The model under review builds one solid part; all positions refer to its coordinate system, in mm. A direction names the side the tool comes from. Give positions to 0.01 mm unless a question says otherwise; leave off trailing zeros. Loops run counter-clockwise (first coordinate to the right, second up) from the corner with the lowest first, then second, coordinate; pieces in that order, holes last. Notation, with made-up numbers: (5.25, -37) - (25.25, -37) arc R7 cw to (25.25, -29) - close; hole circle Ø6 at (82, -28.5). An arc over 180 degrees is marked (long way). Return JSON: item names as keys, results as strings. Group by question number.
from build123d import *

# Parameters (mm, degrees)
SKETCH1_R           = 4.7625
SKETCH1_R_2         = 1.65
BOSS_EXTRUDE1_DEPTH = 15
SKETCH2_R           = 4.7625
BOSS_EXTRUDE2_DEPTH = 15
CUT_EXTRUDE1_REACH  = 66.755
SKETCH3_R           = 2


with BuildPart() as part:
    # Sketch1 → Boss-Extrude1 (new body, symmetric)
    with BuildSketch(Plane.XY):
        with BuildLine():
            Line((-13.253372163, -1.044486042), (-7.531237528, -10.955513958))
            ThreePointArc((-7.531237528, -10.955513958), (-6.784217233, -11.816359568), (-5.770008435, -12.336431676))
            Line((-5.770008435, -12.336431676), (-0.836847118, -13.76941319))
            ThreePointArc((-0.836847118, -13.76941319), (0, -13.888495471), (0.836847118, -13.76941319))
            Line((0.836847118, -13.76941319), (5.770008435, -12.336431676))
            ThreePointArc((5.770008435, -12.336431676), (6.784217233, -11.816359568), (7.531237528, -10.955513958))
            Line((7.531237528, -10.955513958), (13.253372163, -1.044486042))
            ThreePointArc((13.253372163, -1.044486042), (13.625376182, 0.032875315), (13.568667441, 1.171241953))
            Line((13.568667441, 1.171241953), (12.343085176, 6.159975731))
            ThreePointArc((12.343085176, 6.159975731), (12.027789898, 6.944247736), (11.506238058, 7.609437458))
            Line((11.506238058, 7.609437458), (7.798659006, 11.165189723))
            ThreePointArc((7.798659006, 11.165189723), (6.841158949, 11.783484253), (5.722134635, 12))
            Line((5.722134635, 12), (-5.722134635, 12))
            ThreePointArc((-5.722134635, 12), (-6.841158949, 11.783484253), (-7.798659006, 11.165189723))
            Line((-7.798659006, 11.165189723), (-11.506238058, 7.609437458))
            ThreePointArc((-11.506238058, 7.609437458), (-12.027789898, 6.944247736), (-12.343085176, 6.159975731))
            Line((-12.343085176, 6.159975731), (-13.568667441, 1.171241953))
            ThreePointArc((-13.568667441, 1.171241953), (-13.625376182, 0.032875315), (-13.253372163, -1.044486042))
        make_face()
        Circle(SKETCH1_R, mode=Mode.SUBTRACT)
        with Locations((-8.238066653, 4.75625)):
            Circle(SKETCH1_R_2, mode=Mode.SUBTRACT)
        with Locations((8.238066653, 4.75625)):
            Circle(SKETCH1_R_2, mode=Mode.SUBTRACT)
        with Locations((0, -9.5125)):
            Circle(SKETCH1_R_2, mode=Mode.SUBTRACT)
    extrude(amount=BOSS_EXTRUDE1_DEPTH, both=True)

    # Sketch2 → Boss-Extrude2 (add, symmetric)
    with BuildSketch(Plane.XY):
        with BuildLine():
            Line((-12.421472807, 5.666457921), (-9.735682804, 41.826981922))
            ThreePointArc((-9.735682804, 41.826981922), (0, 50.866372944), (9.735682804, 41.826981922))
            Line((9.735682804, 41.826981922), (12.421472807, 5.666457921))
            Line((12.421472807, 5.666457921), (0, 12))
            Line((0, 12), (-12.421472807, 5.666457921))
        make_face()
        with Locations((0, 41.103872944)):
            Circle(SKETCH2_R, mode=Mode.SUBTRACT)
    extrude(amount=BOSS_EXTRUDE2_DEPTH, both=True)

    # Sketch3 → Cut-Extrude1 (cut, up to next)
    with BuildSketch(Plane(origin=(0, 50.866372944, 0), x_dir=(1, 0, 0), z_dir=(0, 1, 0)), mode=Mode.PRIVATE) as cut_extrude1_sk1:
        Circle(SKETCH3_R)
    cut_extrude1_tool1 = extrude(cut_extrude1_sk1.sketch, amount=-CUT_EXTRUDE1_REACH, mode=Mode.PRIVATE) & part.part
    add(cut_extrude1_tool1.solids().sort_by_distance((0, 50.866373, 0))[0], mode=Mode.SUBTRACT)


solid = part.part
Item 1: Take a section at A-A (x = 0). State the section outline as (y, z) points.
Item 2: For P1, Ø5, axis at x = 9.5, z = -1, coming from the +Y side; P2, Ø2, axis at y = 20, z = 7, coming from the +X side; P3, Ø5, axis at x = 1, z = 10, coming from the -Y side; P4, Ø1, axis at y = 26, z = 4, coming from the -X side, all flat-tipped, find the tip position at first contact; note any pin that passes through.
Item 3: For L1, parallel to Y at x = 0, z = 3.5; L2, parallel to Z at x = 0, y = 49.25; L3, parallel to Y at x = 1, z = 11, list the stretches that pass through material, from the lowest coordinate up. Write a range as from..to.
Item 4: Take a section at B-B (z = 0). State how many separate pieces and enclosed holes the cut face has, then the cut area to 3 significant figures.
Item 5: Take a section at D-D (y = 40). State the section outline as (x, z) points, then the cut area to 3 significant figures.
Item 6: Mouldability with a two-part tool opening along Y and no side actions: class faces 3 (the face through (-3.78, -2.9, -0.21)), 4 (the face through (0, 19, 15)), 5 (the face through (-12.978, 3.577, 0.21)) as +Y half, -Y half, draft (parallel to the pull), parting line (faces both ways), or undercut.
Item 7: Tool access review of faces 1 (the face through (13.623, 0.017, 0.21)), 2 (the face through (0, 48, -2)): name each direction out of +Z, -Z, +X, -X, +Y, -Y from which nothing blocks a thin tool from reaching the whole face with its end or side.
Item 8: Take a section at C-C (x = 8.25). State the section outline as (y, z) points, then the cut area to 3 significant figures.
Check sheet entries:
{
 "1": {"outline": "(-13.89, -15) - (-11.16, -15) - (-11.16, 15) - (-13.89, 15) - close; (-7.86, -15) - (-4.76, -15) - (-4.76, 15) - (-7.86, 15) - close; (4.76, -15) - (36.34, -15) - (36.34, 15) - (4.76, 15) - close; (45.87, -15) - (50.87, -15) - (50.87, -2) - (45.87, -2) - close; (45.87, 2) - (50.87, 2) - (50.87, 15) - (45.87, 15) - close"},
 "2": {"P1": "stops at y = 47.91", "P2": "stops at x = 11.43", "P3": "stops at y = -13.89", "P4": "stops at x = -10.95"},
 "3": {"L1": "y = -13.89..-11.16, -7.86..-4.76, 4.76..36.34, 45.87..50.87", "L2": "z = -15..-2, 2..15", "L3": "y = -13.72..-10.82, -8.2..-4.66, 4.66..36.45, 45.76..50.82"},
 "4": {"separate pieces": "1", "enclosed holes": "4", "area": "1,160 mm^2"},
 "5": {"outline": "(-9.87, -15) - (-4.63, -15) - (-4.63, 15) - (-9.87, 15) - close; (4.63, -15) - (9.87, -15) - (9.87, 15) - (4.63, 15) - close", "area": "314 mm^2"},
 "6": {"face 3": "undercut", "face 4": "draft", "face 5": "+Y half"},
 "7": {"face 1": "+Z, -Z, +X", "face 2": "+Y"},
 "8": {"outline": "(-9.71, -15) - (3.11, -15) - (3.11, 15) - (-9.71, 15) - close; (6.41, -15) - (46.32, -15) - (46.32, 15) - (6.41, 15) - close", "area": "1,580 mm^2"}
}
